Can you work these out from the model? Positions are in its coordinate system, mm. A direction names the side the tool comes from. Coordinates: 2 decimals unless noted, no trailing zeros. Write each loop counter-clockwise with the first axis right and the second up, starting at its lowest first coordinate (ties: lowest second). Pieces come first, ordered by that corner, then holes. Notation, with made-up numbers: M 86.25,5 L 127.25,5 A26 cw 127.25,22 Z; hole C 7.5,40.25 d10. An arc over 180 degrees is marked long. Use one line per item in the form item = value. Start each with the question number.
```python
from build123d import *

# Parameters (mm, degrees)
SKETCH_R      = 16.5
SKETCH_R_2    = 4
PAD_DEPTH     = 2
SKETCH001_R   = 6.5
SKETCH001_R_2 = 4
PAD001_DEPTH  = 5
CHAMFER_SIZE  = 1


with BuildPart() as part:
    # Sketch → Pad (new body)
    with BuildSketch(Plane.XY):
        Circle(SKETCH_R)
        Circle(SKETCH_R_2, mode=Mode.SUBTRACT)
    extrude(amount=PAD_DEPTH)

    # Sketch001 (on Face4 of Pad) → Pad001 (join)
    with BuildSketch(Plane.XY.offset(2)):
        Circle(SKETCH001_R)
        Circle(SKETCH001_R_2, mode=Mode.SUBTRACT)
    extrude(amount=PAD001_DEPTH)

    # Chamfer
    chamfer_edges = [part.edges().sort_by_distance(p)[0] for p in [
        (-4, 0, 7),
    ]]
    chamfer(chamfer_edges, length=CHAMFER_SIZE)


solid = part.part
```
1) If we mould it in two halves opening along Y, with no side actions, what happens to faces 3 (the face through (15.24, -6.32, 0.99)), 4 (the face through (2, -5, 7)), 5 (the face through (-0.867, -3.905, 2.958))? For each: +Y half, -Y half, draft (parallel to the pull), parting line (faces both ways), or undercut.
2) Will these pins go through, and if not, where does the flat tip stop? pin 1 Ø3 at (x, z) = (9.5, 3) entering from +Y; pin 2 Ø10 at (x, y) = (-13, 12.5) entering from +Z; pin 3 Ø2 at (x, z) = (-5, 4) entering from +Y.
3) Suppose I cut it at D-D on x = 14.5. Please give me the cut outline in (y, z).
4) Please list where these lines run through material, in increasing order: line 1 (Y direction, x = 0, z = 2.95); line 2 (Y direction, x = 0, z = 1.45); line 3 (Z direction, x = 4, y = 10.5).
5) Suppose I cut it at A-A on y = 0. Please give me the cut outline in (x, z), and give its area (3 significant figures).
6) Suppose I cut it at C-C on z = 4. Please give me the cut outline in (x, y), and give its area (3 significant figures).
7) Which directions (+Z, -Z, +X, -X, +Y, -Y) give clear straight access to the entire face, cutting with the end or side of a thin tool? Please do faces 1 (the face through (-5.158, -3.955, 4.465)), 2 (the face through (3, -3, 0)).
Computed values:
q1.face_3 = parting line
q1.face_4 = draft
q1.face_5 = undercut
q2.pin_1 = 14.21
q2.pin_2 = 2
q2.pin_3 = 5.12
q3.outline = M -7.87,0 L 7.87,0 L 7.87,2 L -7.87,2 Z
q4.line_1 = -6.5 to -4, 4 to 6.5
q4.line_2 = -16.5 to -4, 4 to 16.5
q4.line_3 = 0 to 2
q5.outline = M -16.5,0 L -4,0 L -4,6 L -5,7 L -6.5,7 L -6.5,2 L -16.5,2 Z; M 4,0 L 16.5,0 L 16.5,2 L 6.5,2 L 6.5,7 L 5,7 L 4,6 Z
q5.area = 74.0 mm²
q6.outline = C 0,0 d13; hole C 0,0 d8
q6.area = 82.5 mm²
q7.face_1 = +Z
q7.face_2 = -Z, +X, -X, +Y, -Y
